The listing builds one solid part. Answer for the finished solid, in the listing's coordinates (mm). A direction names the side the tool comes from. Round coordinates to 2 decimals unless told otherwise and drop trailing zeros. Write each loop counter-clockwise with the first axis right and the second up, starting at its lowest first coordinate (ties: lowest second). Pieces come first, ordered by that corner, then holes. Notation, with made-up numbers: M 75,27.5 L 122,27.5 A30 cw 122,53.5 Z; hole C 63,-36 d1. An arc over 180 degrees is marked long. Put each result on its own line as item: value. Start each with the question number.
```python
from build123d import *

# Parameters (mm, degrees)
F0_R     = 25.908
F0_R_2   = 7.5184
F1_DEPTH = 15.494
F2_R     = 11.0109
F3_DEPTH = 10.541
F4_R     = 11.0109
F5_DEPTH = 10.541


with BuildPart() as f1:
    # F0 (on Front) → F1 (new body, symmetric)
    with BuildSketch(Plane.XZ):
        Circle(F0_R)
        Circle(F0_R_2, mode=Mode.SUBTRACT)
    extrude(amount=F1_DEPTH, both=True)

    # F2 (on face) → F3 (cut)
    with BuildSketch(Plane.XZ.offset(15.494)):
        Circle(F2_R)
    extrude(amount=-F3_DEPTH, mode=Mode.SUBTRACT)

    # F4 (on face) → F5 (cut)
    with BuildSketch(Plane(origin=(0, 15.494, 0), x_dir=(-1, 0, 0), z_dir=(0, 1, 0))):
        Circle(F4_R)
    extrude(amount=-F5_DEPTH, mode=Mode.SUBTRACT)

    # F6 (on Right) → F7 (revolve, cut)
    with BuildSketch(Plane.YZ):
        with BuildLine():
            Line((-15.494, 14.4014569813), (-15.494, 14.605))
            ThreePointArc((-15.494, 14.605), (-15.4944077798, 14.5032284906), (-15.494, 14.4014569813))
        make_face()
        with BuildLine():
            ThreePointArc((15.494, 14.4014569813), (15.4944077798, 14.5032284906), (15.494, 14.605))
            Line((15.494, 14.605), (15.494, 14.4014569813))
        make_face()
        with BuildLine():
            Line((-8.382, 25.908), (8.382, 25.908))
            ThreePointArc((8.382, 25.908), (4.2751259826, 27.1166131912), (0, 26.8919848915))
            ThreePointArc((0, 26.8919848915), (-4.2751259826, 27.1166131912), (-8.382, 25.908))
        make_face()
        with BuildLine():
            ThreePointArc((0, 26.8919848915), (4.2751259826, 27.1166131912), (8.382, 25.908))
            ThreePointArc((8.382, 25.908), (13.5435812801, 21.2667533897), (15.494, 14.605))
            Line((15.494, 14.605), (15.494, 30.48))
            Line((15.494, 30.48), (-15.494, 30.48))
            Line((-15.494, 30.48), (-15.494, 14.605))
            ThreePointArc((-15.494, 14.605), (-13.5435812801, 21.2667533897), (-8.382, 25.908))
            ThreePointArc((-8.382, 25.908), (-4.2751259826, 27.1166131912), (0, 26.8919848915))
        make_face()
    revolve(axis=Axis((0, -4.953, 0), (0, 1, 0)), mode=Mode.SUBTRACT)


solid = f1.part
```
Item 1: Section B-B (z = 0) is taken. Give the vertices of the cut face in (x, y) (3 decimals), and give its area (3 significant figures).
Item 2: Section C-C (y = -11) is taken. Give the vertices of the cut face in (x, z), and give its area (3 significant figures).
Item 3: Which of the six approach directions +Z, -Z, +X, -X, +Y, -Y give full straight-line access (tool end or side, diameter ignored) to faces 1 (the cylindrical face through (-1.63, 0.07, -7.34)), 2 (the flat face through (-5, 4.953, -7)), 3 (the cylindrical face through (5.919, -10.297, 9.284))?
Item 4: Section D-D (y = 10.5) is taken. Give the vertices of the cut face in (x, z).
Item 5: Consider line 1 along X through (y, z) = (0.5, 0); line 2 along Y through (x, z) = (-1, -8). Determine where each line is inside the solid, lowest interval first. Write a range as [from, to].
Item 6: Flat-ended cylindrical pins translate along their axes: pin 1 (1.5 mm diameter, centred on x = -10, y = -3, fed in from -Z); pin 2 (20 mm diameter, centred on x = 0, z = 0, fed in from -Y); pin 3 (4 mm diameter, centred on x = 9.5, y = 2.5, fed in from +Z). Find the tip coordinate at first contact, or state that the pin passes through.
Item 7: Determine the mould class of faces 4 (the flat face through (2, 15.494, 11)), 5 (the cylindrical face through (-5.919, 10.297, 9.284)), 6 (the cylindrical face through (24.712, -0.117, 7.782)) for opening direction X: released by +X, released by -X, zero draft, split by the parting line, or undercut.
Item 8: Section A-A (x = 0) is taken. Give the vertices of the cut face in (y, z) (3 decimals).
Output values:
1. outline: M -25.908,-8.382 A12.7 ccw -14.605,-15.494 L -11.011,-15.494 L -11.011,-4.953 L -7.518,-4.953 L -7.518,4.953 L -11.011,4.953 L -11.011,15.494 L -14.605,15.494 A12.7 ccw -25.908,8.382 Z; M 7.518,-4.953 L 11.011,-4.953 L 11.011,-15.494 L 14.605,-15.494 A12.7 ccw 25.908,-8.382 L 25.908,8.382 A12.7 ccw 14.605,15.494 L 11.011,15.494 L 11.011,4.953 L 7.518,4.953 Z
1. area: 900 mm^2
2. outline: C 0,0 d48.39; hole C 0,0 d22.02
2. area: 1,460 mm^2
3. face 1: +Y, -Y
3. face 2: +Y
3. face 3: -Y
4. outline: C 0,0 d49.2; hole C 0,0 d22.02
5. line 1: x = [-25.91, -7.52], [7.52, 25.91]
5. line 2: y = [-4.95, 4.95]
6. pin 1: stops at z = -24.2
6. pin 2: stops at y = -4.95
6. pin 3: stops at z = 24.8
7. face 4: zero draft
7. face 5: undercut
7. face 6: split by the parting line
8. outline: M -15.494,-14.605 A12.7 ccw -8.382,-25.908 L 8.382,-25.908 A12.7 ccw 15.494,-14.605 L 15.494,-11.011 L 4.953,-11.011 L 4.953,-7.518 L -4.953,-7.518 L -4.953,-11.011 L -15.494,-11.011 Z; M -15.494,11.011 L -4.953,11.011 L -4.953,7.518 L 4.953,7.518 L 4.953,11.011 L 15.494,11.011 L 15.494,14.605 A12.7 ccw 8.382,25.908 L -8.382,25.908 A12.7 ccw -15.494,14.605 Z
